The drawing under review shows one solid part. Ordinate dimensions are in mm from its lowest x, y, z. A direction names the side the tool comes from. Coordinates: 2 decimals unless noted, no trailing zeros. Write each loop counter-clockwise with the first axis right and the second up, starting at its lowest first coordinate (ties: lowest second). Pieces come first, ordered by that corner, then holes.
1) We need section B-B on x = 20. Write out the cut boundary in (y, z), then the cut area to 3 significant figures.
2) To check wall thickness, follow line 1 along X through (y, z) = (21.25, 6.5); line 2 along Y through (x, z) = (0.4, 8.5). State the ranges of each line that lie inside material, in increasing order.
3) Insertion check: P1, Ø5, axis at y = 19, z = 4.5, coming from the +X side; P2, Ø5, axis at x = 8, z = 6.5, coming from the +Y side; P3, Ø12, axis at x = 20.5, y = 7.5, coming from the +Z side. Each pin has a flat end and moves straight along its axis. Give the tip position at first contact, or say it passes through.
4) For the marked faces 1 and 2, list the 3-axis set-ups (+Z, -Z, +X, -X, +Y, -Y) from which the entire face can be reached by the end or side of a thin tool; tool diameter is ignored.
5) We need section A-A on y = 21.75. Write out the cut boundary in (x, z).
6) We need section C-C on z = 8.5. Write out the cut boundary in (x, y).
7) We need section D-D on z = 12. Write out the cut boundary in (x, y), then the cut area to 3 significant figures.
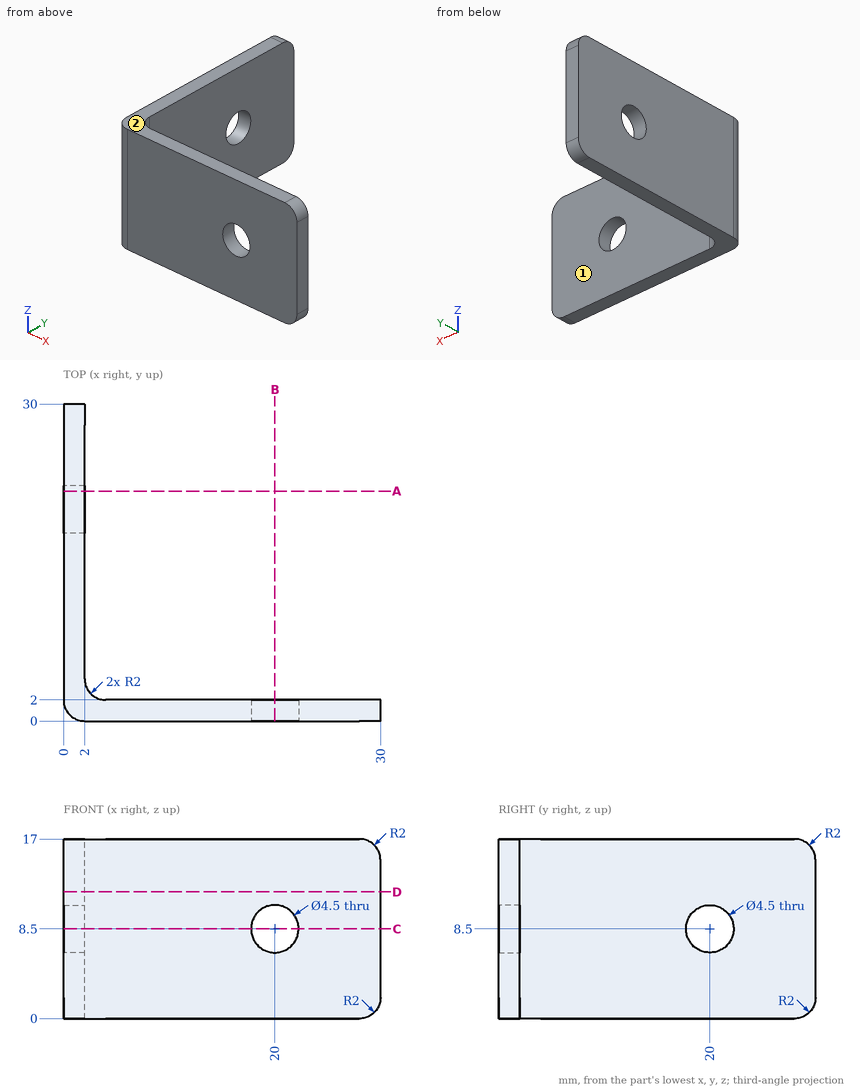
Result:
1. outline: (0, 0) - (2, 0) - (2, 6.25) - (0, 6.25) - close; (0, 10.75) - (2, 10.75) - (2, 17) - (0, 17) - close
1. area: 25.0 mm2
2. line 1: x = 0 to 2
2. line 2: y = 0.8 to 17.75, 22.25 to 30
3. P1: stops at x = 2
3. P2: stops at y = 2
3. P3: stops at z = 17
4. face 1: +Z, -Z, +X, +Y
4. face 2: +Z, +X, -X, +Y, -Y
5. outline: (0, 0) - (2, 0) - (2, 7.09) - (0, 7.09) - close; (0, 9.91) - (2, 9.91) - (2, 17) - (0, 17) - close
6. outline: (0, 2) arc R2 ccw to (2, 0) - (17.75, 0) - (17.75, 2) - (4, 2) arc R2 cw to (2, 4) - (2, 17.75) - (0, 17.75) - close; (0, 22.25) - (2, 22.25) - (2, 30) - (0, 30) - close; (22.25, 0) - (30, 0) - (30, 2) - (22.25, 2) - close
7. outline: (0, 2) arc R2 ccw to (2, 0) - (30, 0) - (30, 2) - (4, 2) arc R2 cw to (2, 4) - (2, 30) - (0, 30) - close
7. area: 116 mm2
